The model under review builds one solid part; all positions refer to its coordinate system, in mm. A direction names the side the tool comes from. Coordinates: 2 decimals unless noted, no trailing zeros. Loops run counter-clockwise (first coordinate to the right, second up) from the corner with the lowest first, then second, coordinate; pieces in that order, holes last. Notation, with made-up numbers: (54, -9.75) -> (94, -9.75) arc R30 cw to (94, 25.25) -> close; hole circle Ø3 at (68.25, 83.5). An arc over 180 degrees is marked (long way). One line per question, with ' | ' between items. Start each with the question number.
from build123d import *

# Parameters (mm, degrees)
ESQUISSE2_W              = 30
ESQUISSE2_H              = 30
BOSS_EXTRU_1_DEPTH       = 5
ESQUISSE16_R             = 2.5
BOSS_EXTRU_7_DEPTH       = 6
CONG_3_R                 = 1
ESQUISSE18_R             = 2.5
BOSS_EXTRU_9_DEPTH       = 6
CONG_5_R                 = 1
ESQUISSE8_R              = 12.5
ENL_V_MAT_EXTRU_1_DEPTH  = 2
ESQUISSE19_R             = 7.5
BOSS_EXTRU_10_DEPTH      = 2
ESQUISSE33_R             = 4
ENL_V_MAT_EXTRU_3_DEPTH  = 6
ESQUISSE35_R             = 2.5
BOSS_EXTRU_26_DEPTH      = 6
CONG_6_R                 = 1
BOSS_EXTRU_27_DEPTH      = 2
BOSS_EXTRU_27_DEPTH_BACK = 5.5


with BuildPart() as part:
    # Esquisse2 → Boss.-Extru.1 (new body)
    with BuildSketch(Plane.XY):
        Rectangle(ESQUISSE2_W, ESQUISSE2_H)
    extrude(amount=BOSS_EXTRU_1_DEPTH)

    # Esquisse16 → Boss.-Extru.7 (add)
    with BuildSketch(Plane.ZY.offset(15)):
        with Locations((2.5, 7)):
            Circle(ESQUISSE16_R)
        with Locations((2.5, -7)):
            Circle(ESQUISSE16_R)
    extrude(amount=BOSS_EXTRU_7_DEPTH)

    # Congé3
    cong_3_edges = [part.edges().sort_by_distance(p)[0] for p in [
        (-21, 7, 0),
        (-21, -7, 0),
    ]]
    fillet(cong_3_edges, radius=CONG_3_R)

    # Esquisse18 → Boss.-Extru.9 (add)
    with BuildSketch(Plane(origin=(15, 0, 0), x_dir=(0, 0, -1), z_dir=(1, 0, 0))):
        with Locations((-2.5, 7)):
            Circle(ESQUISSE18_R)
    extrude(amount=BOSS_EXTRU_9_DEPTH)

    # Congé5
    cong_5_edges = [part.edges().sort_by_distance(p)[0] for p in [
        (21, 7, 5),
    ]]
    fillet(cong_5_edges, radius=CONG_5_R)

    # Esquisse8 → Enlèv. mat.-Extru.1 (cut)
    with BuildSketch(Plane.XY.offset(5)):
        Circle(ESQUISSE8_R)
    extrude(amount=-ENL_V_MAT_EXTRU_1_DEPTH, mode=Mode.SUBTRACT)

    # Esquisse19 → Boss.-Extru.10 (add)
    with BuildSketch(Plane.XY.offset(3)):
        Circle(ESQUISSE19_R)
    extrude(amount=BOSS_EXTRU_10_DEPTH)

    # Esquisse33 → Enlèv. mat.-Extru.3 (cut, through all)
    with BuildSketch(Plane.XY.offset(5)):
        Circle(ESQUISSE33_R)
    extrude(amount=-ENL_V_MAT_EXTRU_3_DEPTH, mode=Mode.SUBTRACT)

    # Esquisse35 → Boss.-Extru.26 (add)
    with BuildSketch(Plane(origin=(0, 15, 0), x_dir=(1, 0, 0), z_dir=(0, 1, 0))):
        with Locations((7, -2.5)):
            Circle(ESQUISSE35_R)
    extrude(amount=BOSS_EXTRU_26_DEPTH)

    # Congé6
    cong_6_edges = [part.edges().sort_by_distance(p)[0] for p in [
        (4.5, 21, 2.5),
    ]]
    fillet(cong_6_edges, radius=CONG_6_R)

    # Esquisse31 → Boss.-Extru.27 (add, two sides)
    with BuildSketch(Plane.XY.offset(3)) as boss_extru_27_sk:
        Polygon((-8.131727984, 10.253048327), (-6.01040764, 12.374368671), (-1.060660172, 7.424621202), (-3.181980515, 5.303300859), align=None)
    extrude(amount=BOSS_EXTRU_27_DEPTH)
    extrude(boss_extru_27_sk.sketch, amount=-BOSS_EXTRU_27_DEPTH_BACK)


solid = part.part
1) Consider section A-A, the plane y = 0. Write out the cut boundary in (x, z).
2) Consider section D-D, the plane x = -12. Write out the cut boundary in (y, z).
3) Mouldability with a two-part tool opening along X and no side actions: class faces 1 (the face through (2.374, -7.114, 3.986)), 2 (the face through (-7.086, 11.299, -1.232)), 3 (the face through (15, -4, 2)) as +X half, -X half, draft (parallel to the pull), parting line (faces both ways), or undercut.
4) Wall thickness on L1, parallel to Y at x = 0, z = 3.35; L2, parallel to Y at x = 0, z = 2.1; L3, parallel to Z at x = 5, y = 6: over which ranges is each line inside the solid? List them lowest first.
5) Consider section C-C, the plane x = -16.5. Write out the cut boundary in (y, z), plus the area to 3 significant figures.
6) Insertion check: pin 1 Ø15 at (x, y) = (1.5, -3.5) entering from -Z; pin 2 Ø1.5 at (y, z) = (12.5, 3.5) entering from -X; pin 3 Ø1.5 at (y, z) = (11, 2.5) entering from +X. Each pin has a flat end and moves straight along its axis. Give the tip position at first contact, or say it passes through.
7) Machinability: for faces 4 (the face through (-5.62, 7.74, -1.23)), 5 (the face through (-2.106, 6.379, -1.232)), 6 (the face through (17, 5, 1)), which of the approach directions +Z, -Z, +X, -X, +Y, -Y give a long, thin tool a straight path to every point of the face, cutting with its end or side? Answer none if there is none.
Filled sheet:
1) outline: (-15, 0) -> (-4, 0) -> (-4, 5) -> (-7.5, 5) -> (-7.5, 3) -> (-12.5, 3) -> (-12.5, 5) -> (-15, 5) -> close; (4, 0) -> (15, 0) -> (15, 5) -> (12.5, 5) -> (12.5, 3) -> (7.5, 3) -> (7.5, 5) -> (4, 5) -> close
2) outline: (-15, 0) -> (15, 0) -> (15, 5) -> (3.5, 5) -> (3.5, 3) -> (-3.5, 3) -> (-3.5, 5) -> (-15, 5) -> close
3) face 1: undercut | face 2: -X half | face 3: +X half
4) L1: -15 to -12.5, -7.5 to -4, 4 to 7.5, 12.5 to 15 | L2: -15 to -4, 4 to 15 | L3: 0 to 3
5) outline: circle Ø5 at (-7, 2.5); circle Ø5 at (7, 2.5) | area: 39.3 mm^2
6) pin 1: z = 0 | pin 2: x = -15 | pin 3: x = 15
7) face 4: -Z, -X, -Y | face 5: -Z, +X, -Y | face 6: +X
